The model under review builds one solid part; all positions refer to its coordinate system, in mm. A direction names the side the tool comes from. Round coordinates to 2 decimals unless told otherwise and drop trailing zeros. Order: outer loops, then holes, each group sorted by start corner. A loop starts at its lowest first (then second) coordinate and runs counter-clockwise, first axis right, second up. Notation, with made-up numbers: M 39.25,-39.5 L 61.25,-39.5 A16 cw 61.25,-20.5 Z; hole C 10.5,48 d5. An arc over 180 degrees is marked long. Use a Markdown table: item, result. Add a question column.
1. To check wall thickness, follow probe 1 along X at (y, z) = (-20.5, -2.5); probe 2 along X at (y, z) = (-15.75, -1.25); probe 3 along Z at (x, y) = (-3, -8.25). State the ranges of each line that lie inside material, in increasing order.
2. Consider section D-D on x = -2.5. State the section outline as (y, z) points.
3. The part is to be moulded in two halves that separate along Z. For faces 1 (the flat face through (2.9, -12.3, 2.5)), 2 (the flat face through (-3.1, -12, 5)), 3 (the flat face through (-2.9, -12.3, 2.5)), 4 (the cylindrical face through (0.9, -12.3, 7.5)), say which applies: +Z half, -Z half, draft (parallel to the pull), parting line (faces both ways), or undercut.
4. Consider section A-A on z = -1. State the section outline as (x, y) points.
5. Insertion check: P1, Ø0.5, axis at y = -11, z = -2.5, coming from the -X side; P2, Ø1.1, axis at y = -13.5, z = 2.5, coming from the +X side. Each pin has a flat end and moves straight along its axis. Give the tip position at first contact, or say it passes through.
6. For faces 5 (the flat face through (0.04, -12.32, 6.57)), 6 (the flat face through (-2, -12, -2)), 7 (the flat face through (2.9, -12.3, -2.5)), 8 (the flat face through (-2.9, -12.3, -2.5)), list the 3-axis set-ups (+Z, -Z, +X, -X, +Y, -Y) from which the entire face can be reached by the end or side of a thin tool; tool diameter is ignored.
7. Consider section C-C on z = 4.75. State the section outline as (x, y) points, then the cut area to 3 significant figures.
from build123d import *

# Parameters (mm, degrees)
F1_DEPTH = 25


with BuildPart() as f1:
    # F0 (on Front) → F1 (new body)
    with BuildSketch(Plane.XZ):
        with BuildLine():
            Line((-2, -7.5), (-2, 3.5))
            ThreePointArc((-2, 3.5), (-0.376864, 3.184528), (0.866667, 4.274356))
            Line((0.866667, 4.274356), (2, 3.5))
            Line((2, 3.5), (2, -7.5))
            Line((2, -7.5), (3.1, -5.5))
            Line((3.1, -5.5), (3.1, -3.5))
            Line((3.1, -3.5), (2.9, -3))
            Line((2.9, -3), (2.9, -2))
            Line((2.9, -2), (3.1, -1.5))
            Line((3.1, -1.5), (3.1, 1.5))
            Line((3.1, 1.5), (2.9, 2))
            Line((2.9, 2), (2.9, 3))
            Line((2.9, 3), (3.1, 3.5))
            Line((3.1, 3.5), (3.1, 4.478163))
            Line((3.1, 4.478163), (2.9, 4.478163))
            Line((2.9, 4.478163), (1.299679, 7.25))
            ThreePointArc((1.299679, 7.25), (0.866667, 7.5), (0.433654, 7.25))
            Line((0.433654, 7.25), (-0.366667, 5.863804))
            ThreePointArc((-0.366667, 5.863804), (-0.866667, 3.997779), (-1.366667, 5.863804))
            Line((-1.366667, 5.863804), (-2.166987, 7.25))
            ThreePointArc((-2.166987, 7.25), (-2.72941, 7.482963), (-3.1, 7))
            Line((-3.1, 7), (-3.1, 3.5))
            Line((-3.1, 3.5), (-2.9, 3))
            Line((-2.9, 3), (-2.9, 2))
            Line((-2.9, 2), (-3.1, 1.5))
            Line((-3.1, 1.5), (-3.1, -1.5))
            Line((-3.1, -1.5), (-2.9, -2))
            Line((-2.9, -2), (-2.9, -3))
            Line((-2.9, -3), (-3.1, -3.5))
            Line((-3.1, -3.5), (-3.1, -5.5))
            Line((-3.1, -5.5), (-2, -7.5))
        make_face()
    extrude(amount=F1_DEPTH)


solid = f1.part
Answer block:
| question | item | result |
|---|---|---|
| 1 | probe 1 | -2.9 to -2, 2 to 2.9 |
| 1 | probe 2 | -3.1 to -2, 2 to 3.1 |
| 1 | probe 3 | -5.68 to -3.25, -1.75 to 1.75, 3.25 to 7.3 |
| 2 | outline | M -25,-6.59 L 0,-6.59 L 0,7.49 L -25,7.49 Z |
| 3 | face 1 | undercut |
| 3 | face 2 | draft |
| 3 | face 3 | undercut |
| 3 | face 4 | +Z half |
| 4 | outline | M -3.1,-25 L -2,-25 L -2,0 L -3.1,0 Z; M 2,-25 L 3.1,-25 L 3.1,0 L 2,0 Z |
| 5 | P1 | x = -2.9 |
| 5 | P2 | x = 2.92 |
| 6 | face 5 | +Z, +Y, -Y |
| 6 | face 6 | -Z, +Y, -Y |
| 6 | face 7 | +X, +Y, -Y |
| 6 | face 8 | -X, +Y, -Y |
| 7 | outline | M -3.1,-25 L -1.84,-25 L -1.84,0 L -3.1,0 Z; M 0.1,-25 L 2.74,-25 L 2.74,0 L 0.1,0 Z |
| 7 | area | 97.6 mm^2 |
